```python
from build123d import *

# Parameters (mm, degrees)
F0_W     = 8
F0_H     = 8
F0_H_2   = 15.5
F0_W_2   = 15.5
F1_DEPTH = 3
F3_D     = 8
F4_R     = 2
F5_DEPTH = 8
F7_D     = 1.5


with BuildPart() as f1:
    # F0 (on Top) → F1 (new body)
    with BuildSketch(Plane.XY):
        Rectangle(F0_W, F0_H)
        with Locations((0, 11.75)):
            Rectangle(F0_W, F0_H_2)
        with Locations((-11.75, 0)):
            Rectangle(F0_W_2, F0_H)
        with Locations((11.75, 0)):
            Rectangle(F0_W_2, F0_H)
        with Locations((0, -11.75)):
            Rectangle(F0_W, F0_H_2)
    extrude(amount=F1_DEPTH)

    # F3 (through all)
    with Locations(Plane(origin=(0, 0, 0), x_dir=(1, 0, 0), z_dir=(0, 0, -1))):
        with Locations((0, 0)):
            Hole(F3_D / 2)

    # F4 (on face) → F5 (join)
    with BuildSketch(Plane.XY.offset(3)):
        with Locations((-16, 0)):
            Circle(F4_R)
        with Locations((-8, 0)):
            Circle(F4_R)
        with Locations((0, -8)):
            Circle(F4_R)
        with Locations((0, -16)):
            Circle(F4_R)
        with Locations((8, 0)):
            Circle(F4_R)
        with Locations((16, 0)):
            Circle(F4_R)
        with Locations((0, 8)):
            Circle(F4_R)
        with Locations((0, 16)):
            Circle(F4_R)
    extrude(amount=F5_DEPTH)

    # F7 (through all)
    with Locations(Plane(origin=(0, 0, 0), x_dir=(1, 0, 0), z_dir=(0, 0, -1))):
        with Locations((-16, 0), (-8, 0), (0, -16), (0, -8), (8, 0), (16, 0), (0, 8), (0, 16)):
            Hole(F7_D / 2)


solid = f1.part
```
Check sheet for the modelled part. Datum: model origin and axes. Units: mm. A direction names the side the tool comes from. Coordinates: 2 decimals unless noted, no trailing zeros. Loops run counter-clockwise (first coordinate to the right, second up) from the corner with the lowest first, then second, coordinate; pieces in that order, holes last.
1) Sectioned sample at B-B (x = 16). Record the boundary of the cut face in (y, z), and give its area (3 significant figures).
2) Gauge pin test, flat ends, axial feed: pin 1 (2.5 mm diameter, centred on x = 13.5, z = 1, fed in from +Y); pin 2 (1.4 mm diameter, centred on x = -16, y = 0, fed in from +Z); pin 3 (2 mm diameter, centred on x = 0, y = -8, fed in from +Z); pin 4 (0.9 mm diameter, centred on x = -10.5, z = 1, fed in from -Y). Record the tip position at first contact, or that the pin passes through.
3) Release check for a two-part mould opening along X. For faces 1 (the face through (-4, -12, 1)), 2 (the face through (1, 16, 11)), 3 (the face through (-15.25, -0.03, 5.58)), 4 (the face through (-3, -3, 3)) record: released by +X, released by -X, zero draft, split by the parting line, or undercut.
4) Sectioned sample at A-A (z = 7.5). Count the separate pieces of the cut face and the enclosed holes in it, and give its area (3 significant figures).
5) Access from +Z, -Z, +X, -X, +Y, -Y to the whole of each face (thin tool, end or side, straight path). Record for faces 5 (the face through (4, -12, 1)), 6 (the face through (-12, 4, 1)), 7 (the face through (0, 10, 7)), 8 (the face through (-12, -4, 1)).
6) Material ranges on probe 1 along Y at (x, z) = (0, 2.5); probe 2 along Y at (x, z) = (-8, 4.25); probe 3 along Y at (x, z) = (-18, 2), recorded low to high.
Check sheet entries:
1. outline: (-4, 0) - (-0.75, 0) - (-0.75, 11) - (-2, 11) - (-2, 3) - (-4, 3) - close; (0.75, 0) - (4, 0) - (4, 3) - (2, 3) - (2, 11) - (0.75, 11) - close
1. area: 39.5 mm2
2. pin 1: stops at y = 4
2. pin 2: passes through
2. pin 3: stops at z = 11
2. pin 4: stops at y = -4
3. face 1: released by -X
3. face 2: zero draft
3. face 3: undercut
3. face 4: undercut
4. separate pieces: 8
4. enclosed holes: 8
4. area: 86.4 mm2
5. face 5: +Z, -Z, +X, -Y
5. face 6: +Z, -Z, -X, +Y
5. face 7: +Z
5. face 8: +Z, -Z, -X, -Y
6. probe 1: y = -19.5 to -16.75, -15.25 to -8.75, -7.25 to -4, 4 to 7.25, 8.75 to 15.25, 16.75 to 19.5
6. probe 2: y = -2 to -0.75, 0.75 to 2
6. probe 3: y = -4 to 4
